from build123d import *

# Parameters (mm, degrees)
F0_W     = 50.8
F0_H     = 25.4
F1_DEPTH = 19.177


with BuildPart() as f1:
    # F0 (on Top) → F1 (new body)
    with BuildSketch(Plane.XY):
        Polygon((942.269583, 485.910804), (-327.730417, 485.910804), (-576.028023, 41.410804), (-327.730417, -403.089196), (942.269583, -403.089196), align=None)
        with Locations((589.601648, -351.892287)):
            Rectangle(F0_W, F0_H, mode=Mode.SUBTRACT)
        with Locations((691.201648, -351.892287)):
            Rectangle(F0_W, F0_H, mode=Mode.SUBTRACT)
        with Locations((589.601648, 438.922962)):
            Rectangle(F0_W, F0_H, mode=Mode.SUBTRACT)
        with Locations((691.201648, 439.756531)):
            Rectangle(F0_W, F0_H, mode=Mode.SUBTRACT)
    extrude(amount=F1_DEPTH)


solid = f1.part
The listing builds one solid part. Answer for the finished solid, in the listing's coordinates (mm). Coordinates: 2 decimals unless noted, no trailing zeros. Loops run counter-clockwise (first coordinate to the right, second up) from the corner with the lowest first, then second, coordinate; pieces in that order, holes last.
1) Find section B-B on y = 369. Write down the section's boundary in (x, z), then the cut area to 3 significant figures.
2) Find section A-A on z = 13.25. Write down the section's boundary in (x, y).
3) Find the intervals of material crossed by L1, parallel to Y at x = 586, z = 10.25; L2, parallel to X at y = 30.5, z = 15.25; L3, parallel to X at y = 156.5, z = 6, in increasing order.
4) Flat-ended cylindrical pins translate along their axes: pin 1 Ø6 at (y, z) = (-114.5, 2.5) entering from -X; pin 2 Ø6 at (x, z) = (-342.5, 11) entering from +Y; pin 3 Ø5 at (y, z) = (-50.5, 16) entering from -X. Find the tip coordinate at first contact, or state that the pin passes through.
5) Find section C-C on y = 161.5. Write down the section's boundary in (x, z), then the cut area to 3 significant figures.
Values:
1. outline: (-393.04, 0) - (942.27, 0) - (942.27, 19.18) - (-393.04, 19.18) - close
1. area: 25,600 mm2
2. outline: (-576.03, 41.41) - (-327.73, -403.09) - (942.27, -403.09) - (942.27, 485.91) - (-327.73, 485.91) - close; hole (564.2, -364.59) - (615, -364.59) - (615, -339.19) - (564.2, -339.19) - close; hole (564.2, 426.22) - (615, 426.22) - (615, 451.62) - (564.2, 451.62) - close; hole (665.8, -364.59) - (716.6, -364.59) - (716.6, -339.19) - (665.8, -339.19) - close; hole (665.8, 427.06) - (716.6, 427.06) - (716.6, 452.46) - (665.8, 452.46) - close
3. L1: y = -403.09 to -364.59, -339.19 to 426.22, 451.62 to 485.91
3. L2: x = -569.93 to 942.27
3. L3: x = -511.74 to 942.27
4. pin 1: stops at x = -490.61
4. pin 2: stops at y = 464.84
4. pin 3: stops at x = -526.08
5. outline: (-508.95, 0) - (942.27, 0) - (942.27, 19.18) - (-508.95, 19.18) - close
5. area: 27,800 mm2
